```python
from build123d import *

# Parameters (mm, degrees)
F0_W     = 63.5
F0_H     = 63.5
F1_DEPTH = 6.35
F2_D     = 5.1054
F2_DEPTH = 4.77
F2_TIP   = 1.5338169022


# Not quite as in the source:
# - a length typed as a fraction of an inch, garbled in the dataset ("3 / 203.2 mm" for 3/8 in), is restored


with BuildPart() as f1:
    # F0 (on Top) → F1 (new body)
    with BuildSketch(Plane.XY):
        Rectangle(F0_W, F0_H)
    extrude(amount=-F1_DEPTH)

    # F2
    with Locations(Plane.XY):
        with Locations((0, -25.4), (21.9970452561, -12.7), (21.9970452561, 12.7), (0, 25.4), (-21.9970452561, -12.7), (-21.9970452561, 12.7)):
            Hole(F2_D / 2, depth=F2_DEPTH)
            with Locations((0, 0, -(F2_DEPTH + F2_TIP / 2))):  # 118° drill point
                Cone(0, F2_D / 2, F2_TIP, mode=Mode.SUBTRACT)


solid = f1.part
```
Geometry: final body of the model. Coordinates: model frame, mm. A direction names the side the tool comes from. Give positions to 0.01 mm unless a question says otherwise; leave off trailing zeros. Loops run counter-clockwise (first coordinate to the right, second up) from the corner with the lowest first, then second, coordinate; pieces in that order, holes last. Notation, with made-up numbers: (2.25, -32) -> (39.25, -32) arc R15 ccw to (39.25, -20) -> close; hole circle Ø8 at (-36, -7.5). An arc over 180 degrees is marked (long way). Return JSON: item names as keys, results as strings.
Item 1: Access query for faces 4 (the cylindrical face through (-1.372, 27.552, -2.418)), 5 (the flat face through (31.75, 0, -3)). Directions: +Z, -Z, +X, -X, +Y, -Y. A direction counts if a zero-diameter tool reaches every point of the face in a straight line with its end or side. Return the directions, or none.
Filled in:
{"face 4": "+Z", "face 5": "+Z, -Z, +X, +Y, -Y"}
Item 2: Mould query, pull axis Y, two halves, no side actions, for faces 1 (the flat face through (0, -31.75, -3)), 2 (the cylindrical face through (-19.447, -12.588, -2.418)), 3 (the flat face through (0, 0, 0)). Classes: released by +Y, released by -Y, zero draft, split by the parting line, or undercut.
Filled in:
{"face 1": "released by -Y", "face 2": "undercut", "face 3": "zero draft"}
Item 3: Line query: line 1 (X direction, y = 12.7, z = -2.6); line 2 (Y direction, x = 0, z = -2); line 3 (X direction, y = 25.4, z = -1.4). Output: solid intervals per line, ascending.
Filled in:
{"line 1": "-31.75 to -24.55, -19.44 to 19.44, 24.55 to 31.75", "line 2": "-31.75 to -27.95, -22.85 to 22.85, 27.95 to 31.75", "line 3": "-31.75 to -2.55, 2.55 to 31.75"}
Item 4: Section A-A, the plane z = -3. Output: boundary loops of the cut face in (x, y).
Filled in:
{"outline": "(-31.75, -31.75) -> (31.75, -31.75) -> (31.75, 31.75) -> (-31.75, 31.75) -> close; hole circle Ø5.11 at (-22, -12.7); hole circle Ø5.11 at (-22, 12.7); hole circle Ø5.11 at (0, -25.4); hole circle Ø5.11 at (0, 25.4); hole circle Ø5.11 at (22, -12.7); hole circle Ø5.11 at (22, 12.7)"}
Item 5: Pin query (flat end, axial travel): P1, Ø4.5, axis at x = -22, y = -12.7, coming from the +Z side; P2, Ø6, axis at x = 0, y = -25.4, coming from the +Z side. Return the tip coordinate at first contact, or that it passes through.
Filled in:
{"P1": "z = -4.95", "P2": "z = 0"}
